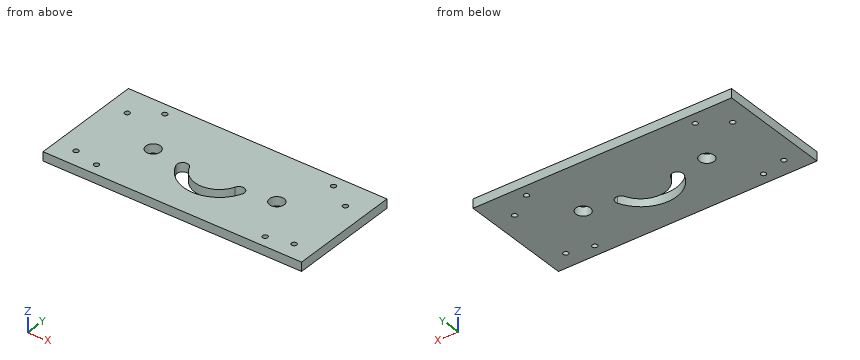
```python
from build123d import *

# Parameters (mm, degrees)
SKETCH1_W           = 230
SKETCH1_H           = 100
SKETCH1_R           = 2.285
SKETCH1_R_2         = 6.5
BOSS_EXTRUDE1_DEPTH = 8


with BuildPart() as part:
    # Sketch1 → Boss-Extrude1 (new body)
    with BuildSketch(Plane.XY):
        Rectangle(SKETCH1_W, SKETCH1_H)
        with Locations((-97, 25)):
            Circle(SKETCH1_R, mode=Mode.SUBTRACT)
        with Locations((-97, -35)):
            Circle(SKETCH1_R, mode=Mode.SUBTRACT)
        with Locations((-75, -40)):
            Circle(SKETCH1_R, mode=Mode.SUBTRACT)
        with Locations(Location((75, -40, 0), (0, 0, 180))):
            Circle(SKETCH1_R, mode=Mode.SUBTRACT)
        with Locations(Location((97, -35, 0), (0, 0, 180))):
            Circle(SKETCH1_R, mode=Mode.SUBTRACT)
        with Locations(Location((97, 25, 0), (0, 0, 180))):
            Circle(SKETCH1_R, mode=Mode.SUBTRACT)
        with Locations((75, 40)):
            Circle(SKETCH1_R, mode=Mode.SUBTRACT)
        with Locations(Location((-75, 40, 0), (0, 0, 180))):
            Circle(SKETCH1_R, mode=Mode.SUBTRACT)
        with Locations((-55, 0)):
            Circle(SKETCH1_R_2, mode=Mode.SUBTRACT)
        with Locations(Location((55, 0, 0), (0, 0, 180))):
            Circle(SKETCH1_R_2, mode=Mode.SUBTRACT)
        with BuildLine():
            ThreePointArc((-29.631019604, -6.885114698), (-0.016046511, -26.820371965), (29.628239655, -6.928730219))
            ThreePointArc((29.628239655, -6.928730219), (26.891929623, -0.408560941), (20.371760345, -3.144870973))
            ThreePointArc((20.371760345, -3.144870973), (-0.008686394, -16.820374674), (-20.368980396, -3.114885302))
            ThreePointArc((-20.368980396, -3.114885302), (-26.885114698, -0.368980396), (-29.631019604, -6.885114698))
        make_face(mode=Mode.SUBTRACT)
    extrude(amount=BOSS_EXTRUDE1_DEPTH)


solid = part.part
```
Can you work these out from the model? Positions are in its coordinate system, mm. Coordinates: 2 decimals unless noted, no trailing zeros. Write each loop counter-clockwise with the first axis right and the second up, starting at its lowest first coordinate (ties: lowest second). Pieces come first, ordered by that corner, then holes. Notation, with made-up numbers: (38, -31.5) - (61, -31.5) arc R20 ccw to (61, -15.5) - close; hole circle Ø5 at (60.25, 20.25). An arc over 180 degrees is marked (long way). Return JSON: item names as keys, results as strings.
Q1. Please list where these lines run through material, in increasing order: L1, parallel to Y at x = 75, z = 3 (3 decimals); L2, parallel to X at y = -0.5, z = 3.5; L3, parallel to X at y = 1, z = 1. Write a range as from..to.
Computed values:
{"L1": "y = -50..-42.285, -37.715..37.715, 42.285..50", "L2": "x = -115..-61.48, -48.52..-27.18, -22.82..22.9, 27.1..48.52, 61.48..115", "L3": "x = -115..-61.42, -48.58..48.58, 61.42..115"}
Q2. If we section it at D-D (z = 1.75): Count the separate pieces of the cut face and the enclosed holes in it, then the cut area to 3 significant figures.
Computed values:
{"separate pieces": "1", "enclosed holes": "11", "area": "21,900 mm2"}
Q3. If we section it at A-A (y = -35): Please give me the cut outline in (x, z) (3 decimals), then the cut area to 3 significant figures.
Computed values:
{"outline": "(-115, 0) - (-99.285, 0) - (-99.285, 8) - (-115, 8) - close; (-94.715, 0) - (94.715, 0) - (94.715, 8) - (-94.715, 8) - close; (99.285, 0) - (115, 0) - (115, 8) - (99.285, 8) - close", "area": "1,770 mm2"}
Q4. If we section it at C-C (x = 25): Please give me the cut outline in (y, z).
Computed values:
{"outline": "(-50, 0) - (-14.8, 0) - (-14.8, 8) - (-50, 8) - close; (-0.04, 0) - (50, 0) - (50, 8) - (-0.04, 8) - close"}
Q5. If we section it at B-B (x = 97): Please give me the cut outline in (y, z) (3 decimals).
Computed values:
{"outline": "(-50, 0) - (-37.285, 0) - (-37.285, 8) - (-50, 8) - close; (-32.715, 0) - (22.715, 0) - (22.715, 8) - (-32.715, 8) - close; (27.285, 0) - (50, 0) - (50, 8) - (27.285, 8) - close"}
